Source: CAD feature listing. Evaluate the final solid. Frame: model axes, mm. A direction names the side the tool comes from. Round coordinates to 2 decimals unless told otherwise and drop trailing zeros. Loops run counter-clockwise (first coordinate to the right, second up) from the corner with the lowest first, then second, coordinate; pieces in that order, holes last. Notation, with made-up numbers: M -8,-15.75 L 28,-15.75 A27 cw 28,20.25 Z; hole C -39,82 d11. An arc over 180 degrees is marked long. Write each question's results on one line, items separated by ' | '. Start each with the question number.
1. Set-up query: faces 5 (the flat face through (77, 10, 2)), 6 (the cylindrical face through (69.612, 7.465, 0.088)). Return all of +Z, -Z, +X, -X, +Y, -Y with unobstructed straight access to the full face (end or side cutting, diameter ignored); none if empty.
2. Section C-C on y = 7.75. Output: boundary loops of the cut face in (x, z).
3. Section B-B on z = 3. Output: boundary loops of the cut face in (x, y).
4. Section D-D on x = 58.5. Output: boundary loops of the cut face in (y, z).
5. Section A-A on y = 2.5. Output: boundary loops of the cut face in (x, z).
6. Ray query, line 1 (Z direction, x = 0, y = 1.4); line 2 (Y direction, x = 68, z = -2.25); line 3 (X direction, y = 0.5, z = 1.25). Return the intervals inside material, ascending.
7. Draft query along X for faces 1 (the flat face through (49, 3, -4)), 2 (the cylindrical face through (98.94, 2.46, -0.09)), 3 (the cylindrical face through (81.61, 7.46, -0.09)), 4 (the cylindrical face through (-4, 2, 0)). Return one class per face: released by +X, released by -X, zero draft, split by the parting line, or undercut.
Autodesk Inventor part; units mm, degrees
ref_plane "YZ Plane" through (0, 0, 0) normal (1, 0, 0) x (0, 1, 0)
ref_plane "XZ Plane" through (0, 0, 0) normal (0, 1, 0) x (-1, 0, 0)
ref_plane "XY Plane" through (0, 0, 0) normal (0, 0, 1) x (1, 0, 0)
sketch "Sketch1" plane through (0, 0, 0) normal (0, 1, 0) x (-1, 0, 0)
  line L0 (0, 0) -> (-96.842, 0) construction
  line L1 (0, 4) -> (-96.842, 4)
  line L2 (-96.842, -4) -> (0, -4)
  arc A0 (0, -4) -> (0, 4) centre (0, 0) ccw
  arc A1 (-96.842, 4) -> (-96.842, -4) centre (-96.842, 0) ccw
  circle A2 centre (0, 0) radius 2.1
  circle A3 centre (-96.842, 0) radius 2.1
  circle A4 centre (-75.611, 0) radius 2.1
  point P0 (-48.421, 0)
  dimension "d0" = 96.842
  dimension "d1" = 8
  dimension "d2" = 4.2
  dimension "d10" = 4.2
  dimension "d28" = 4.2
  dimension "d29" = 75.611
extrude "Extrusion1" add sketch "Sketch1" along normal blind 5
sketch "Sketch4" plane through (0, 5, 0) normal (0, 1, 0) x (1, 0, 0)
  arc A0 (96.842, -4) -> (96.842, 4) centre (96.842, 0) ccw
  line L0 (96.842, 4) -> (0, 4)
  arc A1 (0, 4) -> (0, -4) centre (0, 0) ccw
  line L1 (0, -4) -> (96.842, -4)
  circle A2 centre (75.611, 0) radius 2.1
  circle A3 centre (96.842, 0) radius 2.1
  circle A4 centre (0, 0) radius 2.1
  circle A5 centre (75.611, 0) radius 4
  circle A6 centre (73.611, 0) radius 4
  circle A7 centre (77.611, 0) radius 4
  point P0 (73.611, 4)
  point P1 (73.611, -4)
  point P2 (77.611, -4)
  point P3 (77.611, 4)
  dimension "d30" = 8
  dimension "d31" = 8
  dimension "d32" = 8
  dimension "d33" = 2
  dimension "d34" = 2
extrude "Extrusion7" add sketch "Sketch4" along normal blind 5 contours L1 A5 A7 | A7 A5 | A7 A5 L0 | L1 A6 A5 | A5 A6 A7 | A7 A6 A2 A5 | A5 A6 L0 | A5 A7 A6 | A6 A5 | A5 A6 A7 A2 | A7 A2 A6 | A6 A2 A7 picked at (75.3898, -2.8494) picked at (75.3898, 2.8494)
Taken from the geometry:
1) face 5: +Z, -Z, +X, -X, +Y | face 6: -X, +Y
2) outline: M 73.61,-4 L 77.61,-4 A4 ccw 77.61,4 L 73.61,4 A4 ccw Z; hole C 75.61,0 d4.2
3) outline: M -2.65,0 L 99.49,0 L 99.49,5 L 80.26,5 L 80.26,10 L 70.97,10 L 70.97,5 L -2.65,5 Z
4) outline: M 0,-4 L 5,-4 L 5,4 L 0,4 Z
5) outline: M 0,-4 L 96.84,-4 A4 ccw 96.84,4 L 0,4 A4 ccw Z; hole C 0,0 d4.2; hole C 75.61,0 d4.2; hole C 96.84,0 d4.2
6) line 1: -4 to -2.1, 2.1 to 4 | line 2: 0 to 5 | line 3: -3.8 to -1.69, 1.69 to 73.92, 77.3 to 95.15, 98.53 to 100.64
7) face 1: zero draft | face 2: undercut | face 3: released by +X | face 4: released by -X
